Could you check a few things on this model? Use its own coordinates, in mm. Face numbers are marked on the shaded views. A direction names the side the tool comes from. Give positions to 0.01 mm unless a question says otherwise; leave off trailing zeros. Order: outer loops, then holes, each group sorted by start corner. A loop starts at its lowest first (then second) coordinate and runs counter-clockwise, first axis right, second up.
(1) Imagine slicing it at C-C, the plane x = 0. Write out the boundary of the cut face in (y, z), then the cut area to 3 significant figures.
(2) On a 3-axis mill with a long thin cutter (end or side, diameter ignored), from which of +Z, -Z, +X, -X, +Y, -Y can I reach the whole of each face in a straight line? I mean the marked faces 1, 2, 3, 4 and 5. Say none if no direction works.
(3) If I drill on probe 1 along X at (y, z) = (0, -2.5); probe 2 along Y at (x, z) = (0, -4); probe 3 along X at (y, z) = (-2.25, 4.75), over which ranges is the centre line in solid material (lowest first)?
(4) If we mould it in two halves opening along X, with no side actions, what happens to the marked faces 6, 7 and 8? For each: released by +X, released by -X, zero draft, split by the parting line, or undercut.
(5) Imagine slicing it at A-A, the plane y = -5.25. Write out the boundary of the cut face in (x, z).
(6) Will these pins go through, and if not, where does the flat tip stop? pin 1 (3 mm diameter, centred on y = -6.5, z = -1, fed in from -X); pin 2 (3 mm diameter, centred on y = 2, z = -0.5, fed in from +X); pin 3 (2 mm diameter, centred on x = -7.5, z = -2, fed in from +Y).
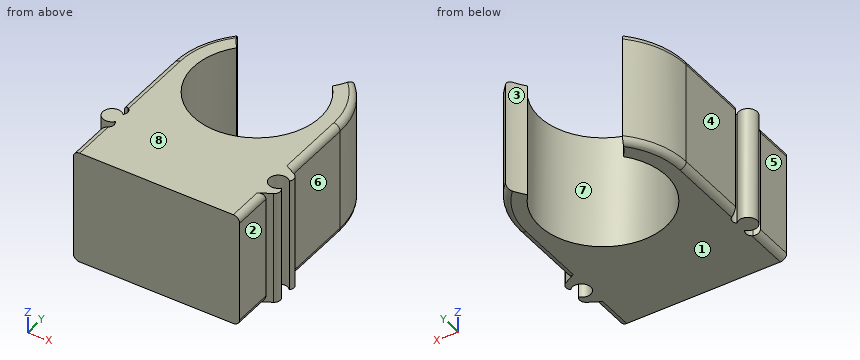
from build123d import *

# Parameters (mm, degrees)
SKETCH1_R            = 7.9375
BOSS_EXTRUDE19_DEPTH = 7.14375
SKETCH2_R            = 7.9375
CUT_EXTRUDE2_DEPTH   = 27.966981115
FILLET6_R            = 0.79375
FILLET7_R            = 0.79375


with BuildPart() as part:
    # Sketch1 → Boss-Extrude19 (new, symmetric)
    with BuildSketch(Plane.XY):
        with BuildLine():
            Line((-10.424745199, -14.070645408), (-10.424745199, -19.05))
            Line((-10.424745199, -19.05), (10.424745199, -19.05))
            Line((10.424745199, -19.05), (10.424745199, -14.070645408))
            Line((10.424745199, -14.070645408), (12.656338894, -12.854690118))
            Line((12.656338894, -12.854690118), (11.297531111, -12.4543891))
            ThreePointArc((11.297531111, -12.4543891), (9.273116661, -11.703061579), (11.297531111, -10.951734059))
            Line((11.297531111, -10.951734059), (12.656338894, -10.551433041))
            Line((12.656338894, -10.551433041), (10.424745199, -9.33547775))
            Line((10.424745199, -9.33547775), (10.424745199, 0))
            ThreePointArc((10.424745199, 0), (0, 10.424745199), (-10.424745199, 0))
            Line((-10.424745199, 0), (-10.424745199, -9.33547775))
            Line((-10.424745199, -9.33547775), (-8.193151504, -10.580610736))
            Line((-8.193151504, -10.580610736), (-9.542093319, -10.963349508))
            ThreePointArc((-9.542093319, -10.963349508), (-11.576373738, -11.703061579), (-9.542093319, -12.442773651))
            Line((-9.542093319, -12.442773651), (-8.193151504, -12.825512422))
            Line((-8.193151504, -12.825512422), (-10.424745199, -14.070645408))
        make_face()
        Circle(SKETCH1_R, mode=Mode.SUBTRACT)
    extrude(amount=BOSS_EXTRUDE19_DEPTH, both=True)

    # Sketch2 → Cut-Extrude2 (cut, through all)
    with BuildSketch(Plane.XY.offset(7.14375)):
        with Locations((0, 10.424745199)):
            Circle(SKETCH2_R)
    extrude(amount=-CUT_EXTRUDE2_DEPTH, mode=Mode.SUBTRACT)

    # Fillet6
    # the kernel refuses this fillet: 0.79375 mm, written as the material it adds along each edge
    with BuildSketch(Plane(origin=(-8.193151504, -12.825512422, -7.14375), x_dir=(-0.8732655856931067, -0.4872445144319999, 0), z_dir=(0, 0, 1))) as fillet6_piece_1:
        with BuildLine():
            CenterArc((1.76022016, -0.79375), FILLET6_R, 90, 104.42604794)
            Line((0.991497097, -0.991497097), (0.976122636, -0.995452039))
            ThreePointArc((0.976122636, -0.995452039), (0.484523228, -0.506973869), (-0.01122532, -0.01122532))
            Line((-0.01122532, -0.01122532), (0, 0.015875))
            Line((0, 0.015875), (1.76022016, 0.015875))
            Line((1.76022016, 0.015875), (1.76022016, 0))
        make_face()
    extrude(amount=14.2875)
    with BuildSketch(Plane(origin=(-8.193151504, -10.580610736, -7.14375), x_dir=(-0.962025917671251, -0.2729581171696266, 0), z_dir=(0, 0, 1))) as fillet6_piece_2:
        with BuildLine():
            CenterArc((1.805929619, -0.683397604), FILLET6_R, 120.57395206, 104.42604794)
            Line((1.244663612, -1.244663612), (1.233438292, -1.255888932))
            Line((1.233438292, -1.255888932), (-0.01122532, -0.01122532))
            Line((-0.01122532, -0.01122532), (0, 0.015875))
            ThreePointArc((0, 0.015875), (0.701094321, 0.015875), (1.394113822, 0.013667952))
            Line((1.394113822, 0.013667952), (1.402188642, 0))
        make_face()
    extrude(amount=14.2875)
    # the kernel refuses this fillet: 0.79375 mm, written as the material it takes off along each edge
    with BuildSketch(Plane(origin=(12.656338894, -12.854690118, -11.562971269), x_dir=(-0.9592408744906186, 0.28258971089987234, 0), z_dir=(0, 0, 1))) as fillet6_2_piece_1:
        with BuildLine():
            CenterArc((1.811210538, 0.688678523), FILLET6_R, 135, 105.183982463)
            Line((1.249944531, 1.249944531), (1.238719211, 1.261169851))
            Line((1.238719211, 1.261169851), (-0.01122532, 0.01122532))
            Line((-0.01122532, 0.01122532), (0, -0.015875))
            ThreePointArc((0, -0.015875), (0.708272458, -0.015875), (1.408651603, -0.01377357))
            Line((1.408651603, -0.01377357), (1.416544915, 0))
        make_face()
    extrude(amount=23.125942539, mode=Mode.SUBTRACT)
    with BuildSketch(Plane(origin=(12.656338894, -10.551433041, -11.562971269), x_dir=(-0.8781068280147701, 0.4784646262722449, 0), z_dir=(0, 0, 1))) as fillet6_2_piece_2:
        with BuildLine():
            CenterArc((1.767688508, 0.79375), FILLET6_R, 164.816017537, 105.183982463)
            Line((1.001648515, 1.001648515), (0.986327716, 1.005806486))
            ThreePointArc((0.986327716, 1.005806486), (0.489598938, 0.512049578), (-0.01122532, 0.01122532))
            Line((-0.01122532, 0.01122532), (0, -0.015875))
            Line((0, -0.015875), (1.767688508, -0.015875))
            Line((1.767688508, -0.015875), (1.767688508, 0))
        make_face()
    extrude(amount=23.125942539, mode=Mode.SUBTRACT)

    # Fillet7
    fillet7_edges = [part.edges().sort_by_distance(p)[0] for p in [
        (-10.424745199, -16.560322704, -7.14375),
        (-10.424745199, -4.667738875, -7.14375),
        (-9.622646342, 4.009986266, -7.14375),
        (9.622646342, 4.009986266, -7.14375),
        (10.424745199, -4.667738875, -7.14375),
        (10.424745199, -16.560322704, -7.14375),
        (10.424745199, -16.560322704, 7.14375),
        (-10.424745199, -16.560322704, 7.14375),
        (-10.424745199, -4.667738875, 7.14375),
        (-9.622646342, 4.009986266, 7.14375),
        (9.622646342, 4.009986266, 7.14375),
        (10.424745199, -4.667738875, 7.14375),
    ]]
    fillet(fillet7_edges, radius=FILLET7_R)


solid = part.part
Answer block:
1. outline: (-19.05, -7.14) - (-7.94, -7.14) - (-7.94, 7.14) - (-19.05, 7.14) - close
1. area: 159 mm2
2. face 1: -Z, +X, -X, +Y, -Y
2. face 2: +Z, -Z, +X, -Y
2. face 3: +Z, -Z, +Y
2. face 4: +Z, -Z, -X, +Y
2. face 5: +Z, -Z, -X, -Y
3. probe 1: x = -10.42 to -7.94, 7.94 to 10.42
3. probe 2: y = -19.05 to -7.94
3. probe 3: x = -10.42 to -7.61, 7.61 to 10.42
4. face 6: released by +X
4. face 7: undercut
4. face 8: zero draft
5. outline: (-10.42, -6.35) arc R0.79 ccw to (-9.63, -7.14) - (-5.95, -7.14) - (-5.95, 7.14) - (-9.63, 7.14) arc R0.79 ccw to (-10.42, 6.35) - close; (5.95, -7.14) - (9.63, -7.14) arc R0.79 ccw to (10.42, -6.35) - (10.42, 6.35) arc R0.79 ccw to (9.63, 7.14) - (5.95, 7.14) - close
6. pin 1: stops at x = -10.42
6. pin 2: stops at x = 10.41
6. pin 3: stops at y = 7.4
